For this review, take the finished solid that the model builds, in its own axes (mm). Round coordinates to 2 decimals unless told otherwise and drop trailing zeros. Order: outer loops, then holes, each group sorted by start corner. A loop starts at its lowest first (then second) coordinate and runs counter-clockwise, first axis right, second up. Notation, with made-up numbers: (48.5, 63.5) - (94.5, 63.5) arc R16 cw to (94.5, 93.5) - close; hole circle Ø10 at (-1, 48). An arc over 180 degrees is marked (long way). One line per item, written item: value.
```python
from build123d import *

# Parameters (mm, degrees)
BASE_FLANGE1_DEPTH  = 50
UNFOLD1_START       = -50
UNFOLD1_DEPTH       = 50
UNFOLD1_2_OUTLINE_W = 3.874357202
UNFOLD1_2_OUTLINE_H = 0.25
UNFOLD1_2_DEPTH     = 50
CUT_EXTRUDE2_DEPTH  = 211.401854511
SKETCH6_W           = 5.069534468
SKETCH6_H           = 3
CUT_EXTRUDE3_DEPTH  = 211.401854511
LPATTERN2_COUNT     = 2
LPATTERN2_PITCH     = 11
SKETCH8_W           = 0.3
SKETCH8_H           = 8
CUT_EXTRUDE4_DEPTH  = 211.401854511
LPATTERN3_COUNT     = 5
LPATTERN3_PITCH     = 11
SKETCH9_W           = 404.874357202
SKETCH9_H           = 46.767764052
CUT_EXTRUDE5_DEPTH  = 211.398245103
FOLD1_START         = -30
FOLD1_OUTLINE_W     = 3.874357202
FOLD1_OUTLINE_H     = 0.25
FOLD1_DEPTH         = 30
FOLD1_START_2       = -22
FOLD1_2_DEPTH       = 3
FOLD1_START_3       = -11
FOLD1_3_DEPTH       = 3
FOLD1_4_DEPTH       = 30
FOLD1_5_DEPTH       = 3
FOLD1_6_DEPTH       = 3
FOLD1_7_DEPTH       = 8
FOLD1_START_4       = -19
FOLD1_8_DEPTH       = 8
FOLD1_START_5       = -8
FOLD1_9_DEPTH       = 8


# Read off the part's stored shape, not the designer's step: Unfold1, Fold1
# Sheet-metal steps are written as plain solids
with BuildPart() as part:
    # Sketch1 → Base-Flange1 (new body)
    with BuildSketch(Plane(origin=(0, 0, 0), x_dir=(1, 0, 0), z_dir=(0, 1, 0))):
        with BuildLine():
            Line((-200.5, 0), (-195.552065744, 0))
            ThreePointArc((-195.552065744, 0), (-195.50012958, -0.001833238), (-195.448451933, -0.007323826))
            Line((-195.448451933, -0.007323826), (-3.868286445, -27.226574518))
            ThreePointArc((-3.868286445, -27.226574518), (0, -27.5), (3.868286445, -27.226574518))
            Line((3.868286445, -27.226574518), (195.448451933, -0.007323826))
            ThreePointArc((195.448451933, -0.007323826), (195.50012958, -0.001833238), (195.552065744, 0))
            Line((195.552065744, 0), (200.5, 0))
            Line((200.5, 0), (200.5, 0.25))
            Line((200.5, 0.25), (195.552065744, 0.25))
            ThreePointArc((195.552065744, 0.25), (195.48250259, 0.247544566), (195.413285693, 0.240190488))
            Line((195.413285692, 0.240190488), (3.833120205, -26.979060204))
            ThreePointArc((3.833120205, -26.979060204), (0, -27.25), (-3.833120205, -26.979060204))
            Line((-3.833120205, -26.979060204), (-195.413285692, 0.240190488))
            ThreePointArc((-195.413285692, 0.240190488), (-195.48250259, 0.247544566), (-195.552065743, 0.25))
            Line((-195.552065744, 0.25), (-200.5, 0.25))
            Line((-200.5, 0.25), (-200.5, 0))
        make_face()
    extrude(amount=-BASE_FLANGE1_DEPTH)

    # Unfold1 outline → Unfold1 (cut)
    with BuildSketch(Plane(origin=(0, 0, 0), x_dir=(1, 0, 0), z_dir=(0, 1, 0)).offset(UNFOLD1_START)):
        with BuildLine():
            Line((195.552065744, 0), (193.722727272, 0))
            Line((193.722727272, 0), (3.833120205, -26.979060204))
            ThreePointArc((3.833120205, -26.979060204), (0, -27.25), (-3.833120205, -26.979060204))
            Line((-3.833120205, -26.979060204), (-193.722727272, 0))
            Line((-193.722727272, 0), (-195.552065744, 0))
            ThreePointArc((-195.552065744, 0), (-195.500129581, -0.001833238), (-195.448451933, -0.007323826))
            Line((-195.448451933, -0.007323826), (-3.868286445, -27.226574518))
            ThreePointArc((-3.868286445, -27.226574518), (0, -27.5), (3.868286445, -27.226574518))
            Line((3.868286445, -27.226574518), (195.448451933, -0.007323826))
            ThreePointArc((195.448451933, -0.007323826), (195.500129581, -0.001833238), (195.552065744, 0))
        make_face()
    extrude(amount=UNFOLD1_DEPTH, mode=Mode.SUBTRACT)

    # Unfold1 2 outline → Unfold1 2 (add)
    with BuildSketch(Plane(origin=(0, 0, 0), x_dir=(1, 0, 0), z_dir=(0, 1, 0)).offset(UNFOLD1_START)):
        with BuildLine():
            ThreePointArc((195.413285692, 0.240190488), (195.48250259, 0.247544566), (195.552065744, 0.25))
            Line((195.552065744, 0.25), (-195.552065744, 0.25))
            ThreePointArc((-195.552065744, 0.25), (-195.48250259, 0.247544566), (-195.413285692, 0.240190488))
            Line((-195.413285692, 0.240190488), (-193.722727272, 0))
            Line((-193.722727272, 0), (193.722727272, 0))
            Line((193.722727272, 0), (195.413285692, 0.240190488))
        make_face()
        with Locations((202.437178601, 0.125)):
            Rectangle(UNFOLD1_2_OUTLINE_W, UNFOLD1_2_OUTLINE_H)
    extrude(amount=UNFOLD1_2_DEPTH)

    # Sketch7 → Cut-Extrude2 (cut, through all)
    with BuildSketch(Plane.XY):
        Polygon((-200.5, -30), (-195.552065744, -30), (1.937178601, -50), (199.304822734, -30), (204.374357202, -30), (227.072555567, -34.066984848), (175.364463115, -76.287353915), (-151.111703925, -76.287353915), (-215.740676819, -64.707357595), align=None)
    extrude(amount=-CUT_EXTRUDE2_DEPTH, mode=Mode.SUBTRACT)

    # Sketch6 → Cut-Extrude3 (cut, through all)
    with BuildSketch(Plane.XY):
        with Locations((-197.965232766, -9.5)):
            Rectangle(SKETCH6_W, SKETCH6_H)
        with Locations((201.839589968, -9.5)):
            Rectangle(SKETCH6_W, SKETCH6_H)
    cut_extrude3 = extrude(amount=-CUT_EXTRUDE3_DEPTH, mode=Mode.SUBTRACT)

    # LPattern2: Cut-Extrude3 ×2
    with Locations(*[(0, -i * LPATTERN2_PITCH, 0) for i in range(1, LPATTERN2_COUNT)]):
        add(cut_extrude3, mode=Mode.SUBTRACT)

    # Sketch8 → Cut-Extrude4 (cut, through all)
    with BuildSketch(Plane.XY):
        with Locations((1.937178601, -4)):
            Rectangle(SKETCH8_W, SKETCH8_H)
    cut_extrude4 = extrude(amount=-CUT_EXTRUDE4_DEPTH, mode=Mode.SUBTRACT)

    # LPattern3: Cut-Extrude4 ×5
    with Locations(*[(0, -i * LPATTERN3_PITCH, 0) for i in range(1, LPATTERN3_COUNT)]):
        add(cut_extrude4, mode=Mode.SUBTRACT)

    # Sketch9 → Cut-Extrude5 (cut, through all)
    with BuildSketch(Plane.XY):
        with Locations((1.937178601, -53.383882026)):
            Rectangle(SKETCH9_W, SKETCH9_H)
    extrude(amount=-CUT_EXTRUDE5_DEPTH, mode=Mode.SUBTRACT)

    # Fold1 outline → Fold1 (cut)
    with BuildSketch(Plane(origin=(0, 0, 0), x_dir=(1, 0, 0), z_dir=(0, 1, 0)).offset(FOLD1_START)):
        with BuildLine():
            Line((193.722727272, 0), (195.413285692, 0.240190488))
            ThreePointArc((195.413285692, 0.240190488), (195.48250259, 0.247544566), (195.552065744, 0.25))
            Line((195.552065744, 0.25), (-195.552065744, 0.25))
            ThreePointArc((-195.552065744, 0.25), (-195.48250259, 0.247544566), (-195.413285692, 0.240190488))
            Line((-195.413285692, 0.240190488), (-193.722727272, 0))
            Line((-193.722727272, 0), (193.722727272, 0))
        make_face()
        with Locations((202.437178601, 0.125)):
            Rectangle(FOLD1_OUTLINE_W, FOLD1_OUTLINE_H)
    extrude(amount=FOLD1_DEPTH, mode=Mode.SUBTRACT)

    # Fold1 2 outline → Fold1 2 (cut)
    with BuildSketch(Plane(origin=(0, 0, 0), x_dir=(1, 0, 0), z_dir=(0, 1, 0)).offset(FOLD1_START_2)):
        with BuildLine():
            ThreePointArc((195.552065744, 0.25), (195.48250259, 0.247544566), (195.413285692, 0.240190488))
            Line((195.413285692, 0.240190488), (195.447411381, 0))
            Line((195.447411381, 0), (199.304822734, 0))
            Line((199.304822734, 0), (199.304822734, 0.25))
            Line((199.304822734, 0.25), (195.552065744, 0.25))
        make_face()
        with BuildLine():
            Line((-195.430465532, 0.119271783), (-195.413285692, 0.240190488))
            ThreePointArc((-195.413285692, 0.240190488), (-195.42187059, 0.241371769), (-195.430465532, 0.242477601))
            Line((-195.430465532, 0.242477601), (-195.430465532, 0.119271783))
        make_face()
    extrude(amount=FOLD1_2_DEPTH, mode=Mode.SUBTRACT)

    # Fold1 3 outline → Fold1 3 (cut)
    with BuildSketch(Plane(origin=(0, 0, 0), x_dir=(1, 0, 0), z_dir=(0, 1, 0)).offset(FOLD1_START_3)):
        with BuildLine():
            ThreePointArc((195.552065744, 0.25), (195.48250259, 0.247544566), (195.413285692, 0.240190488))
            Line((195.413285692, 0.240190488), (195.447411381, 0))
            Line((195.447411381, 0), (199.304822734, 0))
            Line((199.304822734, 0), (199.304822734, 0.25))
            Line((199.304822734, 0.25), (195.552065744, 0.25))
        make_face()
        with BuildLine():
            Line((-195.430465532, 0.119271783), (-195.413285692, 0.240190488))
            ThreePointArc((-195.413285692, 0.240190488), (-195.42187059, 0.241371769), (-195.430465532, 0.242477601))
            Line((-195.430465532, 0.242477601), (-195.430465532, 0.119271783))
        make_face()
    extrude(amount=FOLD1_3_DEPTH, mode=Mode.SUBTRACT)

    # Fold1 4 outline → Fold1 4 (add)
    with BuildSketch(Plane(origin=(0, 0, 0), x_dir=(1, 0, 0), z_dir=(0, 1, 0)).offset(FOLD1_START)):
        with BuildLine():
            Line((195.447411381, 0), (193.722727272, 0))
            Line((193.722727272, 0), (3.833120205, -26.979060204))
            ThreePointArc((3.833120205, -26.979060204), (1.99580633, -27.176814697), (0.149314321, -27.249590919))
            Line((0.149314321, -27.249590919), (0.150684177, -27.499587166))
            ThreePointArc((0.150684177, -27.499587166), (2.014116479, -27.426143273), (3.868286445, -27.226574518))
            Line((3.868286445, -27.226574518), (195.448451933, -0.007323826))
            Line((195.448451933, -0.007323826), (195.447411381, 0))
        make_face()
        with BuildLine():
            Line((-0.150684177, -27.499587166), (-0.149314321, -27.249590919))
            ThreePointArc((-0.149314321, -27.249590919), (-1.99580633, -27.176814697), (-3.833120205, -26.979060204))
            Line((-3.833120205, -26.979060204), (-193.722727272, 0))
            Line((-193.722727272, 0), (-195.430465532, 0))
            Line((-195.430465532, 0), (-195.430465532, 0.119271783))
            Line((-195.430465532, 0.119271783), (-195.448451933, -0.007323826))
            Line((-195.448451933, -0.007323826), (-3.868286445, -27.226574518))
            ThreePointArc((-3.868286445, -27.226574518), (-2.014116479, -27.426143273), (-0.150684177, -27.499587166))
        make_face()
    extrude(amount=FOLD1_4_DEPTH)

    # Fold1 5 outline → Fold1 5 (add)
    with BuildSketch(Plane(origin=(0, 0, 0), x_dir=(1, 0, 0), z_dir=(0, 1, 0)).offset(FOLD1_START_2)):
        with BuildLine():
            Line((0.150684177, -27.499587166), (0.149314321, -27.249590919))
            ThreePointArc((0.149314321, -27.249590919), (0, -27.25), (-0.149314321, -27.249590919))
            Line((-0.149314321, -27.249590919), (-0.150684177, -27.499587166))
            ThreePointArc((-0.150684177, -27.499587166), (0, -27.5), (0.150684177, -27.499587166))
        make_face()
    extrude(amount=FOLD1_5_DEPTH)

    # Fold1 6 outline → Fold1 6 (add)
    with BuildSketch(Plane(origin=(0, 0, 0), x_dir=(1, 0, 0), z_dir=(0, 1, 0)).offset(FOLD1_START_3)):
        with BuildLine():
            Line((0.150684177, -27.499587166), (0.149314321, -27.249590919))
            ThreePointArc((0.149314321, -27.249590919), (0, -27.25), (-0.149314321, -27.249590919))
            Line((-0.149314321, -27.249590919), (-0.150684177, -27.499587166))
            ThreePointArc((-0.150684177, -27.499587166), (0, -27.5), (0.150684177, -27.499587166))
        make_face()
    extrude(amount=FOLD1_6_DEPTH)

    # Fold1 7 outline → Fold1 7 (add)
    with BuildSketch(Plane(origin=(0, 0, 0), x_dir=(1, 0, 0), z_dir=(0, 1, 0)).offset(FOLD1_START)):
        with BuildLine():
            Line((195.552065744, 0), (195.447411381, 0))
            Line((195.447411381, 0), (195.448451933, -0.007323826))
            ThreePointArc((195.448451933, -0.007323826), (195.500129581, -0.001833238), (195.552065744, 0))
        make_face()
        with BuildLine():
            ThreePointArc((-195.552065744, 0), (-195.500129581, -0.001833238), (-195.448451933, -0.007323826))
            Line((-195.448451933, -0.007323826), (-195.447411381, 0))
            Line((-195.447411381, 0), (-195.552065744, 0))
        make_face()
    extrude(amount=FOLD1_7_DEPTH)

    # Fold1 8 outline → Fold1 8 (add)
    with BuildSketch(Plane(origin=(0, 0, 0), x_dir=(1, 0, 0), z_dir=(0, 1, 0)).offset(FOLD1_START_4)):
        with BuildLine():
            Line((195.552065744, 0), (195.447411381, 0))
            Line((195.447411381, 0), (195.448451933, -0.007323826))
            ThreePointArc((195.448451933, -0.007323826), (195.500129581, -0.001833238), (195.552065744, 0))
        make_face()
        with BuildLine():
            ThreePointArc((-195.552065744, 0), (-195.500129581, -0.001833238), (-195.448451933, -0.007323826))
            Line((-195.448451933, -0.007323826), (-195.447411381, 0))
            Line((-195.447411381, 0), (-195.552065744, 0))
        make_face()
    extrude(amount=FOLD1_8_DEPTH)

    # Fold1 9 outline → Fold1 9 (add)
    with BuildSketch(Plane(origin=(0, 0, 0), x_dir=(1, 0, 0), z_dir=(0, 1, 0)).offset(FOLD1_START_5)):
        with BuildLine():
            Line((195.552065744, 0), (195.447411381, 0))
            Line((195.447411381, 0), (195.448451933, -0.007323826))
            ThreePointArc((195.448451933, -0.007323826), (195.500129581, -0.001833238), (195.552065744, 0))
        make_face()
        with BuildLine():
            ThreePointArc((-195.552065744, 0), (-195.500129581, -0.001833238), (-195.448451933, -0.007323826))
            Line((-195.448451933, -0.007323826), (-195.447411381, 0))
            Line((-195.447411381, 0), (-195.552065744, 0))
        make_face()
    extrude(amount=FOLD1_9_DEPTH)


solid = part.part
```
Item 1: For P1, Ø1.5, axis at x = -197.5, y = -2, coming from the +Z side; P2, Ø10, axis at x = 26, y = -14, coming from the -Z side; P3, Ø4, axis at x = 197, y = -15, coming from the +Z side, all flat-tipped, find the tip position at first contact; note any pin that passes through.
Returned:
P1: z = 0
P2: z = 23.12
P3: z = 0.07
Item 2: Take a section at B-B (z = 8.75). Write out the cut boundary in (x, y), plus the area to 3 significant figures.
Returned:
outline: (-133.91, -30) - (-132.14, -30) - (-132.14, 0) - (-133.91, 0) - close; (132.14, -30) - (133.91, -30) - (133.91, 0) - (132.14, 0) - close
area: 107 mm^2
Item 3: Take a section at C-C (x = 123). Write out the cut boundary in (y, z), plus the area to 3 significant figures.
Returned:
outline: (-30, 10.05) - (0, 10.05) - (0, 10.3) - (-30, 10.3) - close
area: 7.58 mm^2
Item 4: Take a section at A-A (y = -26). Write out the cut boundary in (x, z), plus the area to 3 significant figures.
Returned:
outline: (-200.5, -0.25) - (-195.55, -0.25) arc R0.99 ccw to (-195.41, -0.24) - (-3.83, 26.98) arc R27.25 cw to (-0.15, 27.25) - (-0.15, 27.5) arc R27.5 ccw to (-3.87, 27.23) - (-195.45, 0.01) arc R0.74 cw to (-195.55, 0) - (-200.5, 0) - close; (0.15, 27.25) arc R27.25 cw to (3.83, 26.98) - (195.41, -0.24) arc R0.99 ccw to (195.55, -0.25) - (200.5, -0.25) - (200.5, 0) - (195.55, 0) arc R0.74 cw to (195.45, 0.01) - (3.87, 27.23) arc R27.5 ccw to (0.15, 27.5) - close
area: 101 mm^2
Item 5: Wall thickness on line 1 (Z direction, x = 99.5, y = -16.5); line 2 (Z direction, x = 114.5, y = -7.75): over which ranges is each line inside the solid? List them lowest first.
Returned:
line 1: 13.39 to 13.64
line 2: 11.26 to 11.51
